```python
from build123d import *

# Parameters (mm, degrees)
SKETCH3_R          = 1.55
CUT_EXTRUDE1_DEPTH = 17.248076809
SKETCH4_R          = 2.610523844
CUT_EXTRUDE2_DEPTH = 17.248076809
FILLET1_R          = 1
CUT_EXTRUDE3_DEPTH = 3


with BuildPart() as part:
    # Sketch2 → Revolve1 (revolve)
    with BuildSketch(Plane.XY, mode=Mode.PRIVATE) as revolve1_sk:
        Polygon((0, 0), (8, 0), (8, 10), (5, 10), (5, 6), (0, 6), align=None)
    revolve(revolve1_sk.sketch.rotate(Axis((0, 0, 0), (1, 0, 0)), 90), axis=Axis((0, 0, 0), (1, 0, 0)))

    # Sketch3 → Cut-Extrude1 (cut, through all)
    with BuildSketch(Plane.ZY):
        Circle(SKETCH3_R)
    extrude(amount=-CUT_EXTRUDE1_DEPTH, mode=Mode.SUBTRACT)

    # Sketch4 → Cut-Extrude2 (cut, through all)
    with BuildSketch(Plane(origin=(8, 0, 0), x_dir=(0, 0, -1), z_dir=(1, 0, 0))):
        with Locations((0, 10)):
            Circle(SKETCH4_R)
        with Locations((8.660254038, 5)):
            Circle(SKETCH4_R)
        with Locations((8.660254038, -5)):
            Circle(SKETCH4_R)
        with Locations((0, -10)):
            Circle(SKETCH4_R)
        with Locations((-8.660254038, -5)):
            Circle(SKETCH4_R)
        with Locations((-8.660254038, 5)):
            Circle(SKETCH4_R)
    extrude(amount=-CUT_EXTRUDE2_DEPTH, mode=Mode.SUBTRACT)

    # Fillet1
    fillet1_edges = [part.edges().sort_by_distance(p)[0] for p in [
        (6.5, 2.588190451, -9.659258263),
        (6.5, 7.071067812, -7.071067812),
        (6.5, -7.071067812, -7.071067812),
        (6.5, -2.588190451, -9.659258263),
        (6.5, -9.659258263, 2.588190451),
        (6.5, -9.659258263, -2.588190451),
        (6.5, -2.588190451, 9.659258263),
        (6.5, -7.071067812, 7.071067812),
        (6.5, 7.071067812, 7.071067812),
        (6.5, 2.588190451, 9.659258263),
        (6.5, 9.659258263, -2.588190451),
        (6.5, 9.659258263, 2.588190451),
    ]]
    fillet(fillet1_edges, radius=FILLET1_R)

    # Sketch5 → Cut-Extrude3 (cut)
    with BuildSketch(Plane(origin=(8, 0, 0), x_dir=(0, 0, -1), z_dir=(1, 0, 0))):
        Polygon((2.749630657, 1.5875), (0, 3.175), (-2.749630657, 1.5875), (-2.749630657, -1.5875), (0, -3.175), (2.749630657, -1.5875), align=None)
    extrude(amount=-CUT_EXTRUDE3_DEPTH, mode=Mode.SUBTRACT)


solid = part.part
```
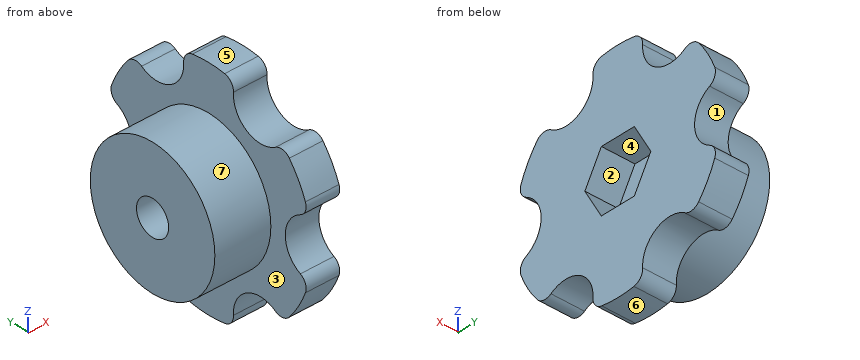
Source: CAD feature listing. Evaluate the final solid. Frame: model axes, mm. Face numbers are marked on the shaded views. A direction names the side the tool comes from. Give positions to 0.01 mm unless a question says otherwise; leave off trailing zeros. Loops run counter-clockwise (first coordinate to the right, second up) from the corner with the lowest first, then second, coordinate; pieces in that order, holes last. Notation, with made-up numbers: (-12.5, -3.75) -> (27.5, -3.75) arc R33 cw to (27.5, 32.25) -> close; hole circle Ø11 at (-38.75, 72.5). An arc over 180 degrees is marked (long way). Put each result on its own line as item: value. Start each with the question number.
1) Cut plane D-D (y = 4.75). Return loops of the section in (x, z), then the cut area to 3 significant figures.
2) Cut plane A-A (y = 0). Return loops of the section in (x, z).
3) Material intervals for probe 1 along Y at (x, z) = (4.25, 0); probe 2 along X at (y, z) = (1.5, -2.25); probe 3 along X at (y, z) = (4.25, -4.5), sorted ascending.
4) Draft query along Z for the marked faces 4, 5, 6 and 7. Return one class per face: released by +Z, released by -Z, zero draft, split by the parting line, or undercut.
5) Contact query for flat-ended pins moving along their axis: P1, Ø2, axis at x = 1.5, y = 0.5, coming from the -Z side; P2, Ø3, axis at x = 6, y = 7, coming from the +Z side; P3, Ø1.9, axis at y = 0, z = 0, coming from the +X side; P4, Ø1, axis at x = 3, y = -2.5, coming from the -Z side. Output: stop coordinate, or through.
6) Cut plane B-B (z = -5.25). Return loops of the section in (x, y).
7) Cut plane C-C (x = 2). Return loops of the section in (y, z).
8) Reachability of the marked faces 1, 2 and 3 from +Z, -Z, +X, -X, +Y, -Y: full face, straight path, thin tool, end or side. Return the list, or none.
Results are:
1. outline: (0, -3.67) -> (5, -3.67) -> (5, -6.06) -> (8, -6.06) -> (8, 6.06) -> (5, 6.06) -> (5, 3.67) -> (0, 3.67) -> close
1. area: 73.0 mm2
2. outline: (0, -6) -> (5, -6) -> (5, -10) -> (8, -10) -> (8, -2.75) -> (5, -2.75) -> (5, -1.55) -> (0, -1.55) -> close; (0, 1.55) -> (5, 1.55) -> (5, 2.75) -> (8, 2.75) -> (8, 10) -> (5, 10) -> (5, 6) -> (0, 6) -> close
3. probe 1: y = -6 to -1.55, 1.55 to 6
3. probe 2: x = 0 to 5
3. probe 3: x = 5 to 8
4. face 4: undercut
4. face 5: released by +Z
4. face 6: released by -Z
4. face 7: split by the parting line
5. P1: stops at z = -6
5. P2: stops at z = 6.66
5. P3: passes through
5. P4: stops at z = -5.66
6. outline: (0, -2.9) -> (5, -2.9) -> (5, -8.51) -> (8, -8.51) -> (8, 8.51) -> (5, 8.51) -> (5, 2.9) -> (0, 2.9) -> close
7. outline: circle Ø12 at (0, 0); hole circle Ø3.1 at (0, 0)
8. face 1: +X, -X, +Y
8. face 2: +X
8. face 3: -X
